Could you check a few things on this model? Use its own coordinates, in mm. A direction names the side the tool comes from. Give positions to 0.01 mm unless a question says otherwise; leave off trailing zeros. Loops run counter-clockwise (first coordinate to the right, second up) from the corner with the lowest first, then second, coordinate; pieces in that order, holes last. Notation, with made-up numbers: (33, 36) - (54, 36) arc R26 ccw to (54, 68) - close; hole circle Ø2 at (75, 76.5). An arc over 180 degrees is marked (long way). Write each question's results on one line, items separated by ' | '. Start each with the question number.
```python
from build123d import *

# Parameters (mm, degrees)
REVOLU_O2_ANGLE          = 180
ESBO_O4_R                = 10
RESSALTO_EXTRUS_O1_DEPTH = 35
RESSALTO_EXTRUS_O2_DEPTH = 20
ESBO_O8_R                = 3.5
CORTE_EXTRUS_O2_DEPTH    = 20
PADR_OCIRCULAR1_COUNT    = 6
ESBO_O6_R                = 3.5
CORTE_EXTRUS_O1_DEPTH    = 15
ESBO_O9_R                = 1.25
CORTE_EXTRUS_O3_DEPTH    = 6
ESBO_O10_W               = 3
ESBO_O10_H               = 120
CORTE_EXTRUS_O4_DEPTH    = 4.5
ESBO_O11_W               = 3
ESBO_O11_H               = 116.4
RESSALTO_EXTRUS_O5_DEPTH = 2
ESBO_O12_R               = 3.25
RESSALTO_EXTRUS_O6_DEPTH = 20
ESBO_O13_R               = 3
RESSALTO_EXTRUS_O7_DEPTH = 20
CORTE_EXTRUS_O5_DEPTH    = 80.8
ESBO_O16_R               = 93
CORTE_EXTRUS_O6_DEPTH    = 10


with BuildPart() as part:
    # Esboço3 → Revolução2 (revolve)
    with BuildSketch(Plane.XY):
        with BuildLine():
            Line((97.5, 79.8), (97.5, 11.304491341))
            Line((97.5, 11.304491341), (97.5, 0))
            Line((97.5, 0), (97.5, -40.2))
            Line((97.5, -40.2), (87.5, -40.2))
            Line((87.5, -40.2), (87.5, 0))
            Line((87.5, 0), (60.342408243, 0))
            Line((60.342408243, 0), (60.342408243, 2.95))
            Line((60.342408243, 2.95), (52, 2.95))
            Line((52, 2.95), (44, 10.95))
            Line((44, 10.95), (31, 10.95))
            Line((31, 10.95), (31, 13.7))
            Line((31, 13.7), (22.6, 13.7))
            Line((22.6, 13.7), (22.6, 17))
            Line((22.6, 17), (19.3, 17))
            Line((19.3, 17), (19.3, 17.7))
            Line((19.3, 17.7), (15.3, 17.7))
            Line((15.3, 17.7), (15.3, 21.05))
            Line((15.3, 21.05), (19.3, 21.05))
            Line((19.3, 21.05), (19.3, 21.2))
            Line((19.3, 21.2), (27.626549127, 25.96))
            Line((27.626549127, 25.96), (31.3, 25.96))
            Line((31.3, 25.96), (31.3, 43.96))
            Line((31.3, 43.96), (32.3, 44.96))
            Line((32.3, 44.96), (38.8, 44.96))
            Line((38.8, 44.96), (38.8, 26.9))
            Line((38.8, 26.9), (55.5, 10.2))
            Line((55.5, 10.2), (83.5, 10.2))
            ThreePointArc((83.5, 10.2), (86.328427125, 11.371572875), (87.5, 14.2))
            Line((87.5, 14.2), (87.5, 76.2))
            Line((87.5, 76.2), (93, 76.2))
            Line((93, 76.2), (93, 79.8))
            Line((93, 79.8), (97.5, 79.8))
        make_face()
    revolve(axis=Axis((0, -3.322055656, 0), (0, 1, 0)), revolution_arc=REVOLU_O2_ANGLE)

    # Esboço4 → Ressalto-extrusão1 (add)
    with BuildSketch(Plane(origin=(0, 79.8, 0), x_dir=(1, 0, 0), z_dir=(0, 1, 0))):
        with Locations((70.71, 70.71)):
            Circle(ESBO_O4_R)
        with Locations((-70.71, 70.71)):
            Circle(ESBO_O4_R)
    extrude(amount=-RESSALTO_EXTRUS_O1_DEPTH)

    # Esboço5 → Ressalto-extrusão2 (add)
    with BuildSketch(Plane.XZ.offset(40.2)):
        with BuildLine():
            Line((10, -105), (10, -96.985823706))
            Line((10, -96.985823706), (-10, -96.985823706))
            Line((-10, -96.985823706), (-10, -105))
            ThreePointArc((-10, -105), (0, -115), (10, -105))
        make_face()
    ressalto_extrus_o2 = extrude(amount=-RESSALTO_EXTRUS_O2_DEPTH)

    # Esboço8 → Corte-extrusão2 (cut)
    with BuildSketch(Plane.XZ.offset(40.2)):
        with Locations((0, -105)):
            Circle(ESBO_O8_R)
    corte_extrus_o2 = extrude(amount=-CORTE_EXTRUS_O2_DEPTH, mode=Mode.SUBTRACT)

    # PadrãoCircular1: Ressalto-extrusão2, Corte-extrusão2 ×6 about axis, 3 skipped
    padr_ocircular1_axis = Axis((0, 0, 0), (0, 1, 0))
    add([ressalto_extrus_o2.rotate(padr_ocircular1_axis, i * 360 / PADR_OCIRCULAR1_COUNT) for i in range(1, PADR_OCIRCULAR1_COUNT) if i not in (2, 3, 4)])
    add([corte_extrus_o2.rotate(padr_ocircular1_axis, i * 360 / PADR_OCIRCULAR1_COUNT) for i in range(1, PADR_OCIRCULAR1_COUNT) if i not in (2, 3, 4)], mode=Mode.SUBTRACT)

    # Esboço6 → Corte-extrusão1 (cut)
    with BuildSketch(Plane(origin=(0, 79.8, 0), x_dir=(1, 0, 0), z_dir=(0, 1, 0))):
        with Locations((70.71, 70.71)):
            Circle(ESBO_O6_R)
        with Locations((-70.71, 70.71)):
            Circle(ESBO_O6_R)
    extrude(amount=-CORTE_EXTRUS_O1_DEPTH, mode=Mode.SUBTRACT)

    # Esboço9 → Corte-extrusão3 (cut)
    with BuildSketch(Plane.XZ.offset(-13.7)):
        with Locations((18.738329701, -18.738329701)):
            Circle(ESBO_O9_R)
        with Locations((-18.738329701, -18.738329701)):
            Circle(ESBO_O9_R)
    extrude(amount=-CORTE_EXTRUS_O3_DEPTH, mode=Mode.SUBTRACT)

    # Esboço10 → Corte-extrusão4 (cut)
    with BuildSketch(Plane.XY):
        with Locations((91.5, 19.8)):
            Rectangle(ESBO_O10_W, ESBO_O10_H)
    extrude(amount=-CORTE_EXTRUS_O4_DEPTH, mode=Mode.SUBTRACT)

    # Esboço11 → Ressalto-extrusão5 (add)
    with BuildSketch(Plane.XY):
        with Locations((-91.5, 18)):
            Rectangle(ESBO_O11_W, ESBO_O11_H)
    extrude(amount=RESSALTO_EXTRUS_O5_DEPTH)

    # Esboço12 → Ressalto-extrusão6 (add)
    with BuildSketch(Plane.XY):
        with BuildLine():
            Line((-100.75, 29.8), (-87.5, 29.8))
            Line((-87.5, 29.8), (-87.5, 9.8))
            Line((-87.5, 9.8), (-100.75, 9.8))
            ThreePointArc((-100.75, 9.8), (-110.75, 19.8), (-100.75, 29.8))
        make_face()
        with Locations((-100.75, 19.8)):
            Circle(ESBO_O12_R, mode=Mode.SUBTRACT)
    extrude(amount=-RESSALTO_EXTRUS_O6_DEPTH)

    # Esboço13 → Ressalto-extrusão7 (add)
    with BuildSketch(Plane.XY):
        with BuildLine():
            Line((100.75, 29.8), (93, 29.8))
            Line((93, 29.8), (93, 9.8))
            Line((93, 9.8), (100.75, 9.8))
            ThreePointArc((100.75, 9.8), (110.75, 19.8), (100.75, 29.8))
        make_face()
        with Locations((100.75, 19.8)):
            Circle(ESBO_O13_R, mode=Mode.SUBTRACT)
    extrude(amount=-RESSALTO_EXTRUS_O7_DEPTH)

    # Esboço14 → Corte-extrusão5 (cut, through all)
    with BuildSketch(Plane(origin=(0, 0, 0), x_dir=(-1, 0, 0), z_dir=(0, -1, 0))):
        with BuildLine():
            ThreePointArc((34.350508428, 67.496062714), (0, 70), (-34.350508428, 67.496062714))
            ThreePointArc((-34.350508428, 67.496062714), (-47.016691783, 50.479370931), (-30, 37.813187576))
            ThreePointArc((-30, 37.813187576), (0, 40), (30, 37.813187576))
            ThreePointArc((30, 37.813187576), (47.016691783, 50.479370931), (34.350508428, 67.496062714))
        make_face()
    extrude(amount=-CORTE_EXTRUS_O5_DEPTH, mode=Mode.SUBTRACT)

    # Esboço16 → Corte-extrusão6 (cut)
    with BuildSketch(Plane(origin=(0, 76.2, 0), x_dir=(1, 0, 0), z_dir=(0, 1, 0))):
        Circle(ESBO_O16_R)
    extrude(amount=CORTE_EXTRUS_O6_DEPTH, mode=Mode.SUBTRACT)


solid = part.part
```
Q1. I want a section at B-B, the plane x = 0. State how many separate pieces and enclosed holes the cut face has, then the cut area to 3 significant figures.
Q2. I'm going to push flat-ended pins straight in: pin 1 Ø8 at (x, y) = (15.5, 24) entering from -Z; pin 2 Ø4 at (x, z) = (-2, -90) entering from +Y; pin 3 Ø11 at (x, z) = (-85, -48.5) entering from +Y; pin 4 Ø6.5 at (y, z) = (-31, -101.5) entering from -X. Where does each tip first touch, or does it pass through?
Q3. I need wall thicknesses on L1, parallel to Z at x = 0, y = -24.5; L2, parallel to X at y = 69, z = -70; L3, parallel to Y at x = -100.75, z = -6.25. Which ranges of each line are inside material? Lowest first, please. Write a range as from..to.
Q4. Which directions (+Z, -Z, +X, -X, +Y, -Y) give clear straight access to the entire face, cutting with the end or side of a thin tool? Please do faces 5 (the face through (-97, 20, 0)), 6 (the face through (99, 9.8, -10)), 7 (the face through (0, 13.7, -23)), 8 (the face through (-82.511, -30.34, -59.185)), 9 (the face through (0, 25.96, -28)).
Q5. I want a section at C-C, the plane z = -90. List the corners of the cut face in (x, y) for me, then the cut area to 3 significant figures.
Q6. If we mould it in two halves opening along Z, with no side actions, what happens to faces 1 (the face through (-0.759, -30.34, -108.417)), 2 (the face through (-71, 64.8, -71)), 3 (the face through (-99, 9.8, -10)), 4 (the face through (55.97, 1.5, -22.55))? For each: +Z half, -Z half, draft (parallel to the pull), parting line (faces both ways), or undercut.
Q7. I want a section at A-A, the plane y = 37. List the corners of the cut face in (x, z) for me, then the cut area to 3 significant figures.
Q8. I want a section at D-D, the plane y = -16.5. List the corners of the cut face in (x, z) for me.
Conclusion:
1) separate pieces: 3 | enclosed holes: 0 | area: 1,980 mm^2
2) pin 1: z = -96.82 | pin 2: y = 76.2 | pin 3: y = 79.8 | pin 4: x = -10
3) L1: -115..-108.5, -101.5..-87.5 | L2: -80.68..-74.14, -67.28..-52.5, 52.5..67.28, 74.14..80.68 | L3: 9.8..16.55, 23.05..29.8
4) face 5: +Z, -X, +Y, -Y | face 6: -Z, +X, -Y | face 7: +Z, -Y | face 8: -Z, +Y, -Y | face 9: +Z, +Y
5) outline: (-37.5, -40.2) - (37.5, -40.2) - (37.5, 79.8) - (23.43, 79.8) - (23.43, 76.2) - (-23.43, 76.2) - (-23.43, 79.8) - (-37.5, 79.8) - close | area: 8,830 mm^2
6) face 1: undercut | face 2: undercut | face 3: draft | face 4: +Z half
7) outline: (-97.5, 0) arc R97.5 ccw to (97.5, 0) - (93, 0) - (93, -4.5) - (90, -4.5) - (90, 0) - (87.5, 0) arc R87.5 cw to (-87.5, 0) - (-90, 0) - (-90, 2) - (-93, 2) - (-93, 0) - close; (-38.8, 0) arc R38.8 ccw to (38.8, 0) - (31.3, 0) arc R31.3 cw to (-31.3, 0) - close | area: 3,720 mm^2
8) outline: (-97.5, 0) arc R97.5 ccw to (97.5, 0) - (93, 0) - (93, -4.5) - (90, -4.5) - (90, 0) - (87.5, 0) arc R87.5 cw to (-87.5, 0) - (-90, 0) - (-90, 2) - (-93, 2) - (-93, 0) - close
